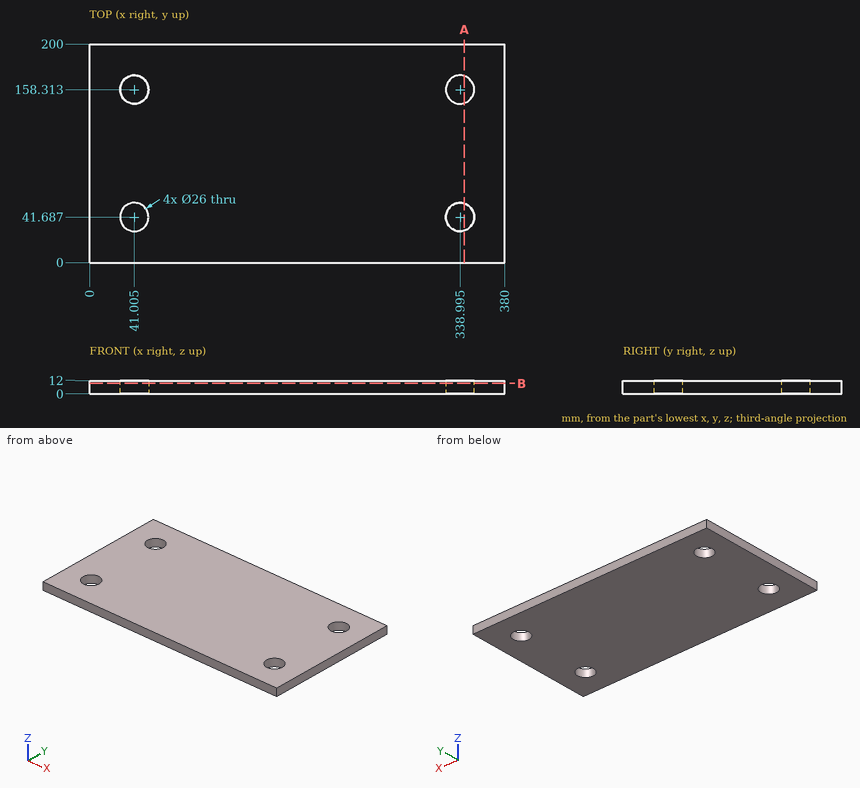
Answer from the drawing. Dimensions are ordinates in mm from the lowest x, y and z of the part. Coordinates: 2 decimals unless noted, no trailing zeros. Write each loop counter-clockwise with the first axis right and the second up, starting at its lowest first coordinate (ties: lowest second). Pieces come first, ordered by that corner, then holes. Notation, with made-up numbers: M 0.25,-15 L 8.25,-15 A21 ccw 8.25,-2 Z; hole C -17.75,34.5 d6. An arc over 180 degrees is marked long. Use a Markdown table: item, result.
Q1. The part is cut by section A-A, the plane x = 343. Write down the section's boundary in (y, z), then the cut area to 3 significant figures.
Answer block:
| item | result |
|---|---|
| outline | M 0,0 L 29.32,0 L 29.32,12 L 0,12 Z; M 54.05,0 L 145.95,0 L 145.95,12 L 54.05,12 Z; M 170.68,0 L 200,0 L 200,12 L 170.68,12 Z |
| area | 1,810 mm2 |
Q2. Straight lines are drawn through the part: L1, parallel to Y at x = 41, z = 9.75; L2, parallel to X at y = 46, z = 3.25; L3, parallel to X at y = 30.5, z = 10.25. For each, find the intervals that lie inside material, in ascending order. Write a range as [from, to].
Answer block:
| item | result |
|---|---|
| L1 | y = [0, 28.69], [54.69, 145.31], [171.31, 200] |
| L2 | x = [0, 28.74], [53.27, 326.73], [351.26, 380] |
| L3 | x = [0, 34.38], [47.63, 332.37], [345.62, 380] |
Q3. The part is cut by section B-B, the plane z = 9.5. Write down the section's boundary in (x, y) (1 decimal), then the cut area to 3 significant figures.
Answer block:
| item | result |
|---|---|
| outline | M 0,0 L 380,0 L 380,200 L 0,200 Z; hole C 41,41.7 d26; hole C 41,158.3 d26; hole C 339,41.7 d26; hole C 339,158.3 d26 |
| area | 73,900 mm2 |
Q4. This flat-tipped pin is pushed along its axis until it touches: pin 1 Ø15.5 at (x, y) = (41, 158.31) entering from -Z. Where does it stop, or does it pass through?
Answer block:
| item | result |
|---|---|
| pin 1 | passes through |
